from build123d import *

# Parameters (mm, degrees)
BOSS_EXTRUDE1_DEPTH = 4.7625
CUT_EXTRUDE2_START  = -6.35
CUT_EXTRUDE2_DEPTH  = 6.35
BOSS_EXTRUDE2_START = 4.7625
SKETCH5_R           = 4.7625
SKETCH5_R_2         = 2.4
BOSS_EXTRUDE2_DEPTH = 4.7625
BOSS_EXTRUDE3_START = 2.38125
BOSS_EXTRUDE3_DEPTH = 2.38125


# Read off the part's stored shape, not the designer's step: Cut-Extrude2
with BuildPart() as part:
    # Sketch1 → Boss-Extrude1 (new, symmetric)
    with BuildSketch(Plane.XY):
        Polygon((0, 0), (-12.7, 0), (-12.7, 3.175), (-23.8125, 3.175), (-23.8125, 6.35), (0, 6.35), align=None)
    extrude(amount=BOSS_EXTRUDE1_DEPTH, both=True)

    # Cut-Extrude2 outline → Cut-Extrude2 (cut)
    with BuildSketch(Plane.XZ.offset(CUT_EXTRUDE2_START)):
        with BuildLine():
            ThreePointArc((0, -1.6e-08), (-1.39490396, -3.367596051), (-4.7625, -4.7625))
            Line((-4.7625, -4.7625), (0, -4.7625))
            Line((0, -4.7625), (0, -1.6e-08))
        make_face()
        with BuildLine():
            ThreePointArc((-4.7625, 4.7625), (-1.394903949, 3.36759604), (0, -1.6e-08))
            Line((0, -1.6e-08), (0, 4.7625))
            Line((0, 4.7625), (-4.7625, 4.7625))
        make_face()
        with BuildLine():
            Line((-23.8125, -4.7625), (-19.05, -4.7625))
            ThreePointArc((-19.05, -4.7625), (-22.417596035, -3.367596056), (-23.8125, -2.9e-08))
            Line((-23.8125, -2.9e-08), (-23.8125, -4.7625))
        make_face()
        with BuildLine():
            Line((-23.8125, 4.7625), (-23.8125, -2.9e-08))
            ThreePointArc((-23.8125, -2.9e-08), (-22.417596056, 3.367596035), (-19.05, 4.7625))
            Line((-19.05, 4.7625), (-23.8125, 4.7625))
        make_face()
    extrude(amount=CUT_EXTRUDE2_DEPTH, mode=Mode.SUBTRACT)

    # Sketch5 → Boss-Extrude2 (add)
    with BuildSketch(Plane(origin=(0, 6.35, 0), x_dir=(1, 0, 0), z_dir=(0, 1, 0)).offset(BOSS_EXTRUDE2_START)):
        with Locations(Location((-19.05, 0, 0), (0, 0, 270))):
            Circle(SKETCH5_R)
        with Locations(Location((-19.05, 0, 0), (0, 0, 90))):
            Circle(SKETCH5_R_2, mode=Mode.SUBTRACT)
    extrude(amount=-BOSS_EXTRUDE2_DEPTH)

    # Sketch6 → Boss-Extrude3 (add)
    with BuildSketch(Plane(origin=(0, 6.35, 0), x_dir=(1, 0, 0), z_dir=(0, 1, 0)).offset(BOSS_EXTRUDE3_START)):
        with BuildLine():
            Line((-19.55, -2.347338919), (-19.55, 2.347338919))
            ThreePointArc((-19.55, 2.347338919), (-19.05, 2.4), (-18.55, 2.347338919))
            Line((-18.55, 2.347338919), (-18.55, -2.347338919))
            ThreePointArc((-18.55, -2.347338919), (-19.05, -2.4), (-19.55, -2.347338919))
        make_face()
    extrude(amount=-BOSS_EXTRUDE3_DEPTH)


solid = part.part
Geometry: final body of the model. Coordinates: model frame, mm. A direction names the side the tool comes from. Give positions to 0.01 mm unless a question says otherwise; leave off trailing zeros. Order: outer loops, then holes, each group sorted by start corner. A loop starts at its lowest first (then second) coordinate and runs counter-clockwise, first axis right, second up. Notation, with made-up numbers: (-22.5, -29) -> (13.5, -29) arc R16 cw to (13.5, -2) -> close; hole circle Ø6 at (-31, -28). An arc over 180 degrees is marked (long way). Answer as a JSON object with one key per item and string values.
Q1. Draft query along X for faces 4 (the flat face through (-12.7, 2, 0)), 5 (the flat face through (-18.55, 8, 0)), 6 (the flat face through (-21, 11.112, 2)). Return one class per face: released by +X, released by -X, zero draft, split by the parting line, or undercut.
Entries:
{"face 4": "released by -X", "face 5": "undercut", "face 6": "zero draft"}
Q2. Section A-A (y = 6.75). State how many separate pieces and enclosed holes the cut face has, plus the area to 3 significant figures.
Entries:
{"separate pieces": "1", "enclosed holes": "2", "area": "57.9 mm^2"}
Q3. Section D-D (y = 1.25). Output: boundary loops of the cut face in (x, z) (1 decimal), plus the area to 3 significant figures.
Entries:
{"outline": "(-12.7, -4.8) -> (-4.8, -4.8) arc R4.8 ccw to (-4.8, 4.8) -> (-12.7, 4.8) -> close", "area": "111 mm^2"}
Q4. Access query for faces 1 (the flat face through (-18, 3.175, 0)), 2 (the flat face through (-6, 0, 0)), 3 (the flat face through (-19, 8.731, 0)). Directions: +Z, -Z, +X, -X, +Y, -Y. A direction counts if a zero-diameter tool reaches every point of the face in a straight line with its end or side. Return the directions, or none.
Entries:
{"face 1": "+Z, -Z, -X, -Y", "face 2": "+Z, -Z, +X, -X, -Y", "face 3": "+Y"}
Q5. Material intervals for probe 1 along X at (y, z) = (8.7, 0); probe 2 along Z at (x, y) = (-19.05, 10.1); probe 3 along X at (y, z) = (9.35, 0), sorted ascending.
Entries:
{"probe 1": "x = -23.81 to -21.45, -19.55 to -18.55, -16.65 to -14.29", "probe 2": "z = -4.76 to -2.4, 2.4 to 4.76", "probe 3": "x = -23.81 to -21.45, -16.65 to -14.29"}
Q6. First-contact query: pin 1 (5 mm diameter, centred on x = -9.5, z = 1.5, fed in from +Y); pin 2 (4 mm diameter, centred on y = 9.5, z = 2, fed in from +X); pin 3 (1 mm diameter, centred on y = 1.5, z = -2, fed in from -X). Flat tips, straight axial feed; report the tip coordinate or a pass-through.
Entries:
{"pin 1": "stops at y = 6.35", "pin 2": "stops at x = -14.29", "pin 3": "stops at x = -12.7"}
